Could you check a few things on this model? Use its own coordinates, in mm. Round coordinates to 2 decimals unless told otherwise and drop trailing zeros. Loops run counter-clockwise (first coordinate to the right, second up) from the corner with the lowest first, then second, coordinate; pieces in that order, holes last. Notation, with made-up numbers: (-20, 32.5) -> (8, 32.5) arc R30 ccw to (8, 68.5) -> close; hole circle Ø8 at (-18.5, 48.25). An arc over 180 degrees is marked (long way). Write each question's results on one line, items separated by ' | '.
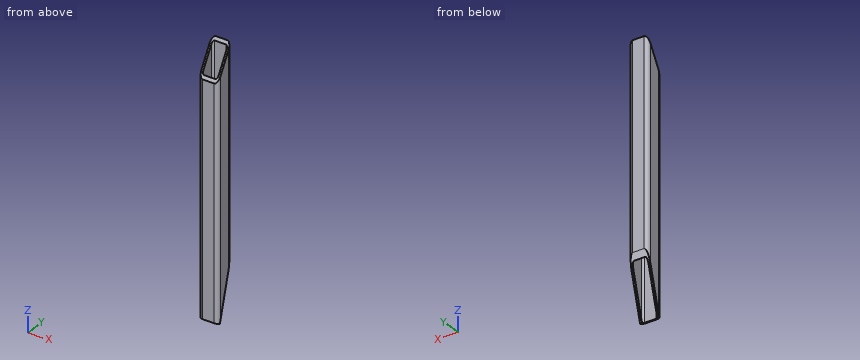
Autodesk Inventor part; units mm, degrees
ref_plane "Start Plane" through (0, 0, 18.432) normal (0, 0, 1) x (1, 0, 0)
ref_plane "End Plane" through (0, 0, 430.8653) normal (0, 0, 1) x (1, 0, 0)
ref_plane "Work Plane4" through (9, -14.4663, 3.9657) normal (0, 0.9644, -0.2644) x (1, 0, 0)
ref_plane "Start Plane" through (0, 0, 18.432) normal (0, 0, 1) x (1, 0, 0)
ref_plane "End Plane" through (0, 0, 430.8653) normal (0, 0, 1) x (1, 0, 0)
sketch "Sketch" plane through (0, 0, 0) normal (0, 0, 1) x (1, 0, 0)
  line L0 (-15, -9) -> (-15, 9)
  line L1 (-9, 15) -> (9, 15)
  line L2 (15, 9) -> (15, -9)
  line L3 (9, -15) -> (-9, -15)
  arc A0 (-15, -9) -> (-9, -15) centre (-9, -9) ccw
  arc A1 (-9, 15) -> (-15, 9) centre (-9, 9) ccw
  arc A2 (15, 9) -> (9, 15) centre (9, 9) ccw
  arc A3 (9, -15) -> (15, -9) centre (9, -9) ccw
  arc A4 (-9, 12) -> (-12, 9) centre (-9, 9) ccw
  line L4 (-9, 12) -> (9, 12)
  arc A5 (12, 9) -> (9, 12) centre (9, 9) ccw
  line L5 (12, 9) -> (12, -9)
  arc A6 (9, -12) -> (12, -9) centre (9, -9) ccw
  line L6 (9, -12) -> (-9, -12)
  arc A7 (-12, -9) -> (-9, -12) centre (-9, -9) ccw
  line L7 (-12, -9) -> (-12, 9)
  line L8 (0, 22.7397) -> (0, -22.7397) construction
  line L9 (-22.7397, 0) -> (22.7397, 0) construction
  dimension "d7" = 6
  dimension "d10" = 30
  dimension "d11" = 30
  dimension "d12" = 3
  dimension "d15" = 15
  dimension "d16" = 15
extrude "Body" add sketch "Sketch" along normal up to surface (412.4333 mm away) from surface at 18.432
sketch "Sketch3" plane through (0, 0, 0) normal (0, 0, 1) x (1, 0, 0)
  line L0 (0, 0) -> (10, 0)
ref_plane "Work Plane3" through (0, 0, 0) normal (0, -1, 0) x (1, 0, 0)
ref_plane "Work Plane4" through (9, -14.4663, 3.9657) normal (0, 0.9644, -0.2644) x (1, 0, 0)
split "Split1" plane through (9, -14.4663, 3.9657) removes the side toward (0, 0.9644, -0.2644)
ref_plane "Work Plane5" through (-9, 3.9657, 14.4663) normal (0, -0.2644, -0.9644) x (1, 0, 0)
split "Split2" plane through (-9, 3.9657, 14.4663) removes the side toward (0, -0.2644, -0.9644)
ref_plane "Work Plane6" through (-9, -208.9131, 53.1585) normal (0, -0.8602, 0.5099) x (1, 0, 0)
split "Split3" plane through (-9, -208.9131, 53.1585) removes the side toward (0, -0.8602, 0.5099)
sketch "Sketch4" plane through (0, 0, 0) normal (0, -1, 0) x (1, 0, 0)
  line L0 (-2, 18.432) -> (12, 18.432)
  line L1 (-2, 430.8653) -> (12, 430.8653)
  dimension "d18" = 412.4333
equation "\"d7\" = G_IR"
equation "\"d10\" = G_H"
equation "\"d11\" = G_W"
equation "\"d12\" = G_T"
equation "\"d15\" = 0.5 * d10"
equation "\"d16\" = 0.5 * d11"
equation "\"d3\" = G_L"
equation "\"G_W\" = 30"
equation "\"G_H\" = 30"
equation "\"G_T\" = 3"
equation "\"G_IR\" = 6"
equation "\"G_L\" = d18"
equation "\"G_OFFSET_START\" = -18.432"
equation "\"G_OFFSET_END\" = -4.11204"
equation "\"d13\" = -G_OFFSET_START"
equation "\"d14\" = G_OFFSET_END + B_L"
equation "\"B_L\" = 434.9773"
properties part number "DIN EN 10219-2 - 30 x 30 x 3  - 412.43" material "Steel, Mild"
1) I want a section at B-B, the plane z = 134. Write out the boundary of the cut face in (x, y), plus the area to 3 significant figures.
Model answer:
outline: (-15, -9) arc R6 ccw to (-9, -15) -> (9, -15) arc R6 ccw to (15, -9) -> (15, 9) arc R6 ccw to (9, 15) -> (-9, 15) arc R6 ccw to (-15, 9) -> close; hole (-12, -9) arc R3 ccw to (-9, -12) -> (9, -12) arc R3 ccw to (12, -9) -> (12, 9) arc R3 ccw to (9, 12) -> (-9, 12) arc R3 ccw to (-12, 9) -> close | area: 301 mm2
2) I want a section at C-C, the plane y = 0.5. Write out the boundary of the cut face in (x, z), plus the area to 3 significant figures.
Model answer:
outline: (-15, 58.56) -> (-12, 58.56) -> (-12, 406.44) -> (-15, 406.44) -> close; (12, 58.56) -> (15, 58.56) -> (15, 406.44) -> (12, 406.44) -> close | area: 2,090 mm2
3) I need wall thicknesses on line 1 (X direction, y = 5, z = 103); line 2 (Y direction, x = -8.5, z = 63). Which ranges of each line are inside material? Lowest first, please.
Model answer:
line 1: x = -15 to -12, 12 to 15 | line 2: y = -15 to -12
4) I'm going to push flat-ended pins straight in: pin 1 (2 mm diameter, centred on x = 2.5, y = 9.5, fed in from -Z); pin 2 (12 mm diameter, centred on x = 2.5, y = -7.5, fed in from -Z); pin 3 (12 mm diameter, centred on x = 0, y = 10, fed in from +Z). Where does each tip first touch, or does it pass through?
Model answer:
pin 1: passes through | pin 2: stops at z = 18.84 | pin 3: stops at z = 430.87
